Part print with two shaded views. Sizes in mm from the minimum x, y, z corner. Give positions to 0.01 mm unless a question says otherwise; leave off trailing zeros. Loops run counter-clockwise (first coordinate to the right, second up) from the corner with the lowest first, then second, coordinate; pieces in that order, holes last. Notation, with made-up numbers: M 17,3.5 L 35,3.5 A37 ccw 35,40.5 Z; hole C 42.25,27 d1. An arc over 180 degrees is marked long. Answer as a JSON object with one key per item and string values. Group by question number.
1. Slice it at A-A (x = 0.4). Give the number of separate pieces and of enclosed holes in the cut face, then the cut area to 3 significant figures.
2. Drill centre lines: line 1 along Z through (x, y) = (0.4, 6); line 2 along Y through (x, z) = (1.95, 4.75) (1 decimal); line 3 along X through (y, z) = (6.5, 4). Where is each one in solid material? Low to high. Write a range as [from, to].
3. Mould opens along Z. For the marked faces 1, 2, 3 and 4 say: released by +Z, released by -Z, zero draft, split by the parting line, or undercut.
4. Slice it at B-B (z = 5.55). List the corners of the cut face in (x, y) (1 decimal).
5. Drop flat-ended pins along their axis: pin 1 Ø4.5 at (y, z) = (6, 15.6) entering from +X (1 decimal); pin 2 Ø4 at (y, z) = (5, 14.5) entering from +X (1 decimal); pin 3 Ø1.5 at (x, z) = (1, 9) entering from +Y. Give the stop position or say it passes through.
6. Slice it at C-C (y = 10.75). List the corners of the cut face in (x, z) (1 decimal).
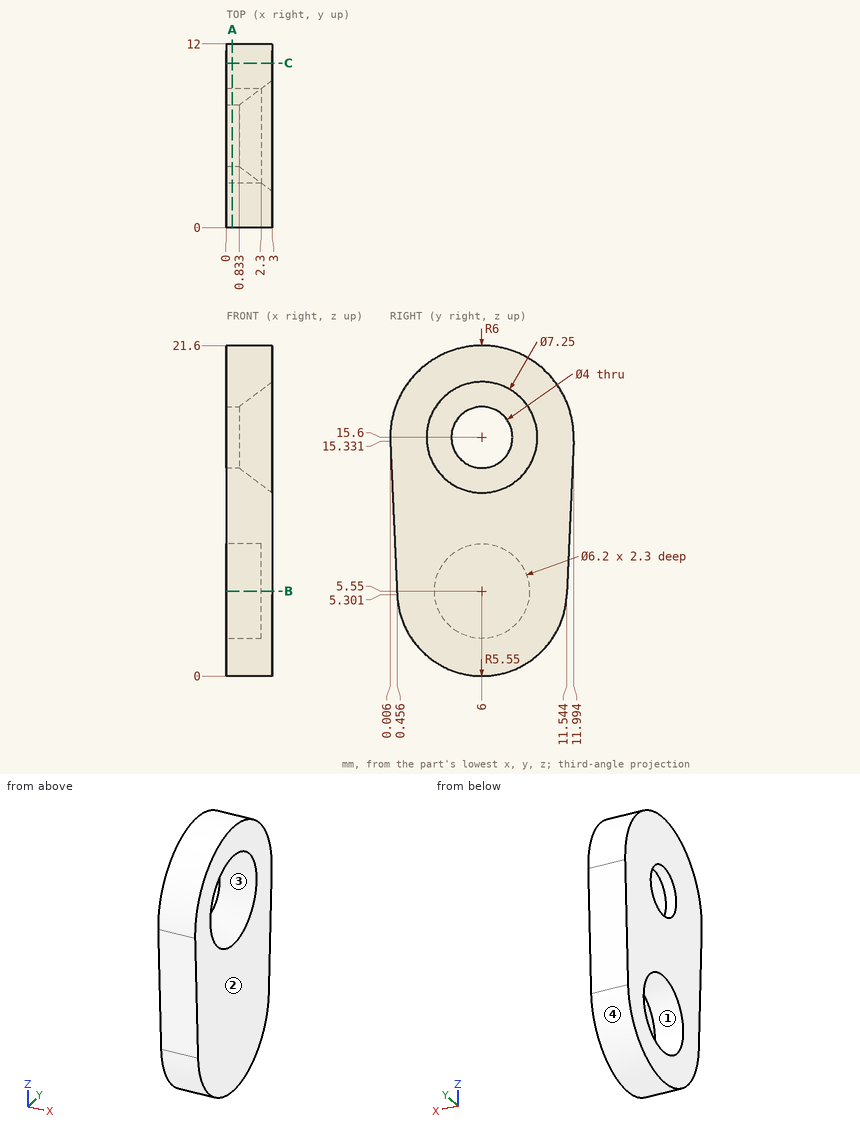
Established:
{
 "1": {"separate pieces": "1", "enclosed holes": "2", "area": "178 mm^2"},
 "2": {"line 1": "z = [0, 2.45], [8.65, 13.6], [17.6, 21.6]", "line 2": "y = [0.5, 3], [9, 11.5]", "line 3": "x = [2.3, 3]"},
 "3": {"face 1": "undercut", "face 2": "zero draft", "face 3": "undercut", "face 4": "released by -Z"},
 "4": {"outline": "M 0,0.4 L 3,0.4 L 3,11.6 L 0,11.6 L 0,9.1 L 2.3,9.1 L 2.3,2.9 L 0,2.9 Z"},
 "5": {"pin 1": "stops at x = 1.2", "pin 2": "stops at x = 2.8", "pin 3": "stops at y = 11.74"},
 "6": {"outline": "M 0,2.7 L 3,2.7 L 3,19.3 L 0,19.3 Z"}
}
